```python
from build123d import *

# Parameters (mm, degrees)
BOSS_EXTRUDE1_DEPTH      = 7
BOSS_EXTRUDE2_START      = 1
SKETCH2_R                = 5
BOSS_EXTRUDE2_DEPTH      = 1
SKETCH3_W                = 5
SKETCH3_H                = 1
F_4_0_4_DIAMETER_HOLE1_D = 4


with BuildPart() as part:
    # Sketch1 → Boss-Extrude1 (new body)
    with BuildSketch(Plane(origin=(0, 0, 74), x_dir=(-1, 0, 0), z_dir=(0, 0, -1))):
        with BuildLine():
            Line((-9.792858273, 22.023664764), (-18.163987442, 36.890703242))
            ThreePointArc((-18.163987442, 36.890703242), (-25.418865109, 42.641693781), (-24.263539525, 33.456250682))
            Line((-24.263539525, 33.456250682), (-15.892410356, 18.589212204))
            ThreePointArc((-15.892410356, 18.589212204), (-16.346796769, 18.007963525), (-16.757092444, 17.394795929))
            Line((-16.757092444, 17.394795929), (-18.965700238, 17.831555144))
            ThreePointArc((-18.965700238, 17.831555144), (-19.514808102, 17.55458812), (-19.379909826, 16.954560925))
            Line((-19.379909826, 16.954560925), (-17.910889228, 15.715657441))
            Line((-17.910889228, 15.715657441), (-17.664910308, 15.504807423))
            ThreePointArc((-17.664910308, 15.504807423), (-17.827013037, 15.010242888), (-17.963165175, 14.507914341))
            Line((-17.963165175, 14.507914341), (-20.19864203, 14.240799695))
            ThreePointArc((-20.19864203, 14.240799695), (-20.635287125, 13.80770474), (-20.32157264, 13.278730827))
            Line((-20.32157264, 13.278730827), (-18.541608797, 12.554415925))
            Line((-18.541608797, 12.554415925), (-18.242512703, 12.429897308))
            ThreePointArc((-18.242512703, 12.429897308), (-18.243852713, 11.909445986), (-18.218113034, 11.389629824))
            Line((-18.218113034, 11.389629824), (-20.261634899, 10.444788361))
            ThreePointArc((-20.261634899, 10.444788361), (-20.543075361, 9.897959827), (-20.081253227, 9.491818847))
            Line((-20.081253227, 9.491818847), (-18.164581401, 9.352993516))
            Line((-18.164581401, 9.352993516), (-17.841645743, 9.32699505))
            ThreePointArc((-17.841645743, 9.32699505), (-17.682091866, 8.831602343), (-17.496979948, 8.345181793))
            Line((-17.496979948, 8.345181793), (-19.148512665, 6.815101178))
            ThreePointArc((-19.148512665, 6.815101178), (-19.247199139, 6.208066452), (-18.682475725, 5.964514314))
            Line((-18.682475725, 5.964514314), (-16.816713109, 6.424767746))
            Line((-16.816713109, 6.424767746), (-16.501549079, 6.499834341))
            ThreePointArc((-16.501549079, 6.499834341), (-16.196719559, 6.077992739), (-15.870355447, 5.672582033))
            Line((-15.870355447, 5.672582033), (-16.968235486, 3.707037218))
            ThreePointArc((-16.968235486, 3.707037218), (-16.874507855, 3.099217089), (-16.262162222, 3.042094373))
            Line((-16.262162222, 3.042094373), (-14.62994266, 4.056373754))
            Line((-14.62994266, 4.056373754), (-14.353400709, 4.22515737))
            ThreePointArc((-14.353400709, 4.22515737), (-13.933134384, 3.918159668), (-13.497464871, 3.633443231))
            Line((-13.497464871, 3.633443231), (-13.934224085, 1.424835437))
            ThreePointArc((-13.934224085, 1.424835437), (-13.657257061, 0.875727573), (-13.057229867, 1.010625848))
            Line((-13.057229867, 1.010625848), (-11.818326382, 2.479646446))
            Line((-11.818326382, 2.479646446), (-11.607476364, 2.725625367))
            ThreePointArc((-11.607476364, 2.725625367), (-11.112911829, 2.563522638), (-10.610583282, 2.427370499))
            Line((-10.610583282, 2.427370499), (-10.343468637, 0.191893645))
            ThreePointArc((-10.343468637, 0.191893645), (-9.910373682, -0.24475145), (-9.381399768, 0.068963034))
            Line((-9.381399768, 0.068963034), (-8.657084866, 1.848926878))
            Line((-8.657084866, 1.848926878), (-8.532566249, 2.148022972))
            ThreePointArc((-8.532566249, 2.148022972), (-8.012114927, 2.146682961), (-7.492298765, 2.17242264))
            Line((-7.492298765, 2.17242264), (-6.547457302, 0.128900776))
            ThreePointArc((-6.547457302, 0.128900776), (-6.000628768, -0.152539686), (-5.594487788, 0.309282448))
            Line((-5.594487788, 0.309282448), (-5.455662457, 2.225954274))
            Line((-5.455662457, 2.225954274), (-5.429663991, 2.548889932))
            ThreePointArc((-5.429663991, 2.548889932), (-4.934271284, 2.708443809), (-4.447850734, 2.893555727))
            Line((-4.447850734, 2.893555727), (-2.917770119, 1.24202301))
            ThreePointArc((-2.917770119, 1.24202301), (-2.310735394, 1.143336536), (-2.067183255, 1.70805995))
            Line((-2.067183255, 1.70805995), (-2.527436687, 3.573822566))
            Line((-2.527436687, 3.573822566), (-2.602503283, 3.888986596))
            ThreePointArc((-2.602503283, 3.888986596), (-2.18066168, 4.193816116), (-1.775250975, 4.520180228))
            Line((-1.775250975, 4.520180228), (0.19029384, 3.422300189))
            ThreePointArc((0.19029384, 3.422300189), (0.79811397, 3.51602782), (0.855236686, 4.128373453))
            Line((0.855236686, 4.128373453), (-0.159042695, 5.760593015))
            Line((-0.159042695, 5.760593015), (-0.327826311, 6.037134965))
            ThreePointArc((-0.327826311, 6.037134965), (-0.020828609, 6.457401291), (0.263887828, 6.893070804))
            Line((0.263887828, 6.893070804), (2.472495622, 6.45631159))
            ThreePointArc((2.472495622, 6.45631159), (3.021603486, 6.733278614), (2.88670521, 7.333305808))
            Line((2.88670521, 7.333305808), (1.417684612, 8.572209293))
            Line((1.417684612, 8.572209293), (1.171705692, 8.783059311))
            ThreePointArc((1.171705692, 8.783059311), (1.333808421, 9.277623846), (1.469960559, 9.779952393))
            Line((1.469960559, 9.779952393), (3.705437414, 10.047067038))
            ThreePointArc((3.705437414, 10.047067038), (4.142082509, 10.480161993), (3.828368024, 11.009135907))
            Line((3.828368024, 11.009135907), (2.048404181, 11.733450809))
            Line((2.048404181, 11.733450809), (1.749308087, 11.857969426))
            ThreePointArc((1.749308087, 11.857969426), (1.750648097, 12.378420747), (1.724908418, 12.89823691))
            Line((1.724908418, 12.89823691), (3.768430283, 13.843078373))
            ThreePointArc((3.768430283, 13.843078373), (4.049870744, 14.389906907), (3.588048611, 14.796047887))
            Line((3.588048611, 14.796047887), (1.671376785, 14.934873217))
            Line((1.671376785, 14.934873217), (1.348441127, 14.960871684))
            ThreePointArc((1.348441127, 14.960871684), (1.188887249, 15.45626439), (1.003775332, 15.942684941))
            Line((1.003775332, 15.942684941), (2.655308048, 17.472765555))
            ThreePointArc((2.655308048, 17.472765555), (2.753994523, 18.079800281), (2.189271109, 18.32335242))
            Line((2.189271109, 18.32335242), (0.323508493, 17.863098988))
            Line((0.323508493, 17.863098988), (0.008344463, 17.788032392))
            ThreePointArc((0.008344463, 17.788032392), (-0.296485057, 18.209873994), (-0.622849169, 18.6152847))
            Line((-0.622849169, 18.6152847), (0.47503087, 20.580829515))
            ThreePointArc((0.47503087, 20.580829515), (0.381303238, 21.188649645), (-0.231042394, 21.245772361))
            Line((-0.231042394, 21.245772361), (-1.863261956, 20.23149298))
            Line((-1.863261956, 20.23149298), (-2.139803907, 20.062709363))
            ThreePointArc((-2.139803907, 20.062709363), (-2.560070232, 20.369707066), (-2.995739745, 20.654423502))
            Line((-2.995739745, 20.654423502), (-2.558980531, 22.863031297))
            ThreePointArc((-2.558980531, 22.863031297), (-2.835947555, 23.412139161), (-3.43597475, 23.277240885))
            Line((-3.43597475, 23.277240885), (-4.674878234, 21.808220287))
            Line((-4.674878234, 21.808220287), (-4.885728252, 21.562241367))
            ThreePointArc((-4.885728252, 21.562241367), (-5.380292787, 21.724344095), (-5.882621334, 21.860496234))
            Line((-5.882621334, 21.860496234), (-6.149735979, 24.095973089))
            ThreePointArc((-6.149735979, 24.095973089), (-6.582830934, 24.532618183), (-7.111804848, 24.218903699))
            Line((-7.111804848, 24.218903699), (-7.83611975, 22.438939856))
            Line((-7.83611975, 22.438939856), (-7.960638367, 22.139843762))
            ThreePointArc((-7.960638367, 22.139843762), (-8.879420123, 22.123890361), (-9.792858273, 22.023664764))
        make_face()
    extrude(amount=-BOSS_EXTRUDE1_DEPTH)

    # Sketch2 → Boss-Extrude2 (add)
    with BuildSketch(Plane(origin=(0, 0, 74), x_dir=(-1, 0, 0), z_dir=(0, 0, -1)).offset(BOSS_EXTRUDE2_START)):
        with Locations((-22.965684708, 38.284870865)):
            Circle(SKETCH2_R)
    extrude(amount=-BOSS_EXTRUDE2_DEPTH)

    # Sketch3 → Revolve1 (revolve)
    with BuildSketch(Plane(origin=(0, 12.143933367, 0), x_dir=(1, 0, 0), z_dir=(0, 1, 0))):
        with Locations((10.746602308, -73.5)):
            Rectangle(SKETCH3_W, SKETCH3_H)
    revolve(axis=Axis((8.246602308, 12.143933367, 73), (0, 0, 1)))

    # Ø4.0 (4) Diameter Hole1 (through all)
    with Locations(Plane.XY.offset(81)):
        with Locations((22.965684708, 38.284870865), (8.246602308, 12.143933367)):
            Hole(F_4_0_4_DIAMETER_HOLE1_D / 2)


solid = part.part
```
Geometry check sheet. Reference: the model listing, model coordinates, mm. A direction names the side the tool comes from. Give positions to 0.01 mm unless a question says otherwise; leave off trailing zeros. Order: outer loops, then holes, each group sorted by start corner. A loop starts at its lowest first (then second) coordinate and runs counter-clockwise, first axis right, second up.
1. Gauge pin test, flat ends, axial feed: pin 1 Ø3.5 at (x, y) = (8.25, 12.14) entering from +Z; pin 2 Ø6.5 at (x, y) = (22.97, 38.28) entering from -Z; pin 3 Ø1.5 at (x, z) = (9, 79) entering from +Y; pin 4 Ø1 at (y, z) = (22.5, 79.5) entering from +X. Record the tip position at first contact, or that the pin passes through.
2. Section check D-D, the plane x = 26. Enter the section's corners in (y, z).
3. Section check C-C, the plane z = 76.75. Give the number of separate pieces and of enclosed holes in the cut face, and give its area (3 significant figures).
4. Section check A-A, the plane x = 12.5. Enter the section's corners in (y, z), and give its area (3 significant figures).
5. Release check for a two-part mould opening along X. For faces 1 (the face through (16.34, 18.02, 77.45)), 2 (the face through (-1.33, 9.27, 77.45)), 3 (the face through (3.694, 2.079, 77.451)), 4 (the face through (20.545, 9.907, 77.451)) record: pulls with the +X half, pulls with the -X half, needs draft (parallel to the pull), parting line crosses it, or undercut.
6. Thickness scan on L1, parallel to X at y = 4, z = 76.5; L2, parallel to Z at x = 4, y = 22; L3, parallel to X at y = 22.5, z = 76.25. Record the ranges inside material, lowest first.
7. Access from +Z, -Z, +X, -X, +Y, -Y to the whole of each face (thin tool, end or side, straight path). Record for faces 5 (the face through (10, 19, 74)), 6 (the face through (0.082, 19.584, 77.451)), 7 (the face through (5.37, 21.72, 77.45)), 8 (the face through (16.2, 6.08, 77.45)), 9 (the face through (10.48, 1.33, 77.45)).
8. Section check B-B, the plane y = 35.5. Enter the section's corners in (x, z), and give its area (3 significant figures).
Values follow:
1. pin 1: passes through
1. pin 2: stops at z = 73
1. pin 3: stops at y = 22.14
1. pin 4: stops at x = 18.38
2. outline: (34.31, 73) - (42.26, 73) - (42.26, 81) - (34.31, 81) - close
3. separate pieces: 1
3. enclosed holes: 2
3. area: 537 mm2
4. outline: (1.67, 74) - (9.52, 74) - (9.52, 73) - (14.77, 73) - (14.77, 74) - (26.83, 74) - (26.83, 81) - (1.67, 81) - close
4. area: 181 mm2
5. face 1: undercut
5. face 2: pulls with the -X half
5. face 3: undercut
5. face 4: pulls with the +X half
6. L1: x = -0.91 to 0.84, 2.44 to 14.05, 14.72 to 16.8
6. L2: z = 74 to 81
6. L3: x = 2.63 to 4.09, 5.96 to 7.81, 10.06 to 18.09
7. face 5: -Z
7. face 6: +Z, -Z, -X
7. face 7: +Z, -Z, +Y
7. face 8: +Z, -Z
7. face 9: +Z, -Z, -Y
8. outline: (17.38, 74) - (18.81, 74) - (18.81, 73) - (27.12, 73) - (27.12, 81) - (17.38, 81) - close
8. area: 76.5 mm2
